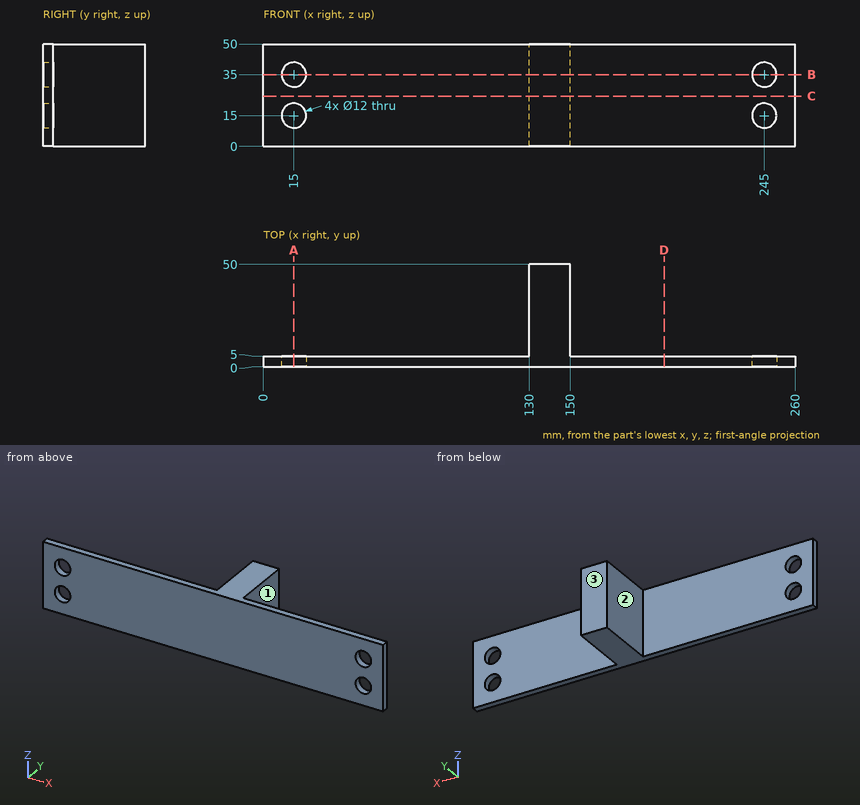
Geometry check sheet. Reference: drawing and pictorial views, mm from the part's lowest x, y, z. A direction names the side the tool comes from. Give positions to 0.01 mm unless a question says otherwise; leave off trailing zeros. Write each loop counter-clockwise with the first axis right and the second up, starting at its lowest first coordinate (ties: lowest second). Pieces come first, ordered by that corner, then holes. Notation, with made-up numbers: M 56,39.5 L 67,39.5 A14 cw 67,47.5 Z; hole C 72,46.5 d10. An arc over 180 degrees is marked long. Use CSV: the item, a comma, the result in double quotes.
1) Cross-section at B-B (z = 35). Enter the section's corners in (x, y).
Final values:
outline,"M 0,0 L 9,0 L 9,5 L 0,5 Z; M 21,0 L 239,0 L 239,5 L 150,5 L 150,50 L 130,50 L 130,5 L 21,5 Z; M 251,0 L 260,0 L 260,5 L 251,5 Z"
2) Material ranges on line 1 along Z through (x, y) = (245, 3); line 2 along Y through (x, z) = (180, 6.5); line 3 along X through (y, z) = (42.5, 9), recorded low to high.
Final values:
line 1,"0 to 9, 21 to 29, 41 to 50"
line 2,"0 to 5"
line 3,"130 to 150"
3) Cross-section at D-D (x = 196). Enter the section's corners in (y, z).
Final values:
outline,"M 0,0 L 5,0 L 5,50 L 0,50 Z"
4) Cross-section at A-A (x = 15). Enter the section's corners in (y, z).
Final values:
outline,"M 0,0 L 5,0 L 5,9 L 0,9 Z; M 0,21 L 5,21 L 5,29 L 0,29 Z; M 0,41 L 5,41 L 5,50 L 0,50 Z"
5) Go/stop test with flat-tipped pins: pin 1 Ø4 at (x, z) = (161, 23) entering from +Y; pin 2 Ø12 at (y, z) = (35.5, 28) entering from -X; pin 3 Ø1.5 at (y, z) = (37, 26.5) entering from +X. Record where each tip stops, or that it passes through.
Final values:
pin 1,"y = 5"
pin 2,"x = 130"
pin 3,"x = 150"
6) Cross-section at C-C (z = 24.5). Enter the section's corners in (x, y), plus the area to 3 significant figures.
Final values:
outline,"M 0,0 L 260,0 L 260,5 L 150,5 L 150,50 L 130,50 L 130,5 L 0,5 Z"
area,"2,200 mm²"
7) Access from +Z, -Z, +X, -X, +Y, -Y to the whole of each face (thin tool, end or side, straight path). Record for the marked faces 1, 2 and 3.
Final values:
face 1,"+Z, -Z, +X, +Y"
face 2,"+Z, -Z, -X, +Y"
face 3,"+Z, -Z, +X, -X, +Y"
